Autodesk Inventor part; units mm, degrees
ref_plane "Work Plane1" through (-12.197, 0, 0) normal (0, -0.8660254, -0.5) x (1, 0, 0)
ref_plane "YZ Plane" through (0, 0, 0) normal (1, 0, 0) x (0, 1, 0)
ref_plane "XZ Plane" through (0, 0, 0) normal (0, 1, 0) x (-1, 0, 0)
sketch "Sketch1" plane through (0, 0, 0) normal (1, 0, 0) x (0, 1, 0)
  line L0 (-6.4231, 0) -> (-3.2116, 5.5626)
  line L1 (-3.2116, 5.5626) -> (3.2116, 5.5626)
  line L2 (3.2116, 5.5626) -> (6.4231, 0)
  line L3 (6.4231, 0) -> (3.2116, -5.5626)
  line L4 (3.2116, -5.5626) -> (-3.2116, -5.5626)
  line L5 (-3.2116, -5.5626) -> (-6.4231, 0)
  point P0 (0, 0)
  point P1 (0, 0)
  dimension "d0" = 12.8463
extrude "Body" add sketch "Sketch1" along normal blind 5.7404
sketch "Sketch2" plane through (0, 0, 0) normal (0, 0, 1) x (1, 0, 0)
  line L0 (0, 3.2116) -> (0, 6.4231)
  line L1 (0, 6.4231) -> (5.7404, 6.4231)
  line L2 (5.7404, 3.2116) -> (5.7404, 6.4231)
  line L3 (-1.1481, 0) -> (6.8885, 0)
  line L4 (0.4968, 6.4231) -> (0, 5.5626)
  line L5 (5.2436, 6.4231) -> (5.7404, 5.5626)
  dimension "d3" = 30
  dimension "d4" = 30
  dimension "d5" = 11.1252
  dimension "d6" = 11.1252
revolve "Chamfer1" cut sketch "Sketch2" angle 360 about axis through (-10, 0, 0) along (1, 0, 0)
sketch "Sketch3" plane through (5.7404, 0, 0) normal (1, 0, 0) x (0, 0, -1)
  arc A0 (-2.7813, -4.8174) -> (2.7813, -4.8174) centre (0, 0) ccw
hole "Thread" at (5.7404, 0, 0) direction (-1, 0, 0) diameter 4.9784 end through all
chamfer "Chamfer2" distance 0.6874 angle 30 1 edges at (5.7404, 0, 2.4892) measured on face at (5.7404, -4.5118, -0.1)
chamfer "Chamfer3" distance 0.6874 angle 30 1 edges at (0, 0, 2.4892) measured on face at (0, -4.5118, -0.1)
ref_plane "Work Plane1" through (-12.197, 0, 0) normal (0, -0.8660254, -0.5) x (1, 0, 0)
equation "\"d0\" = 1.1547 * SW"
equation "\"d1\" = KOH"
equation "\"d3\" = ANG1"
equation "\"d4\" = ANG2"
equation "\"d5\" = SW0"
equation "\"d6\" = SW01"
equation "\"d8\" = -0.5 * GD1 + 0.5 * NND"
equation "\"d40\" = -0.5 * GD1 + 0.5 * NND"
equation "\"d10\" = -0.5 * GD1 + 0.5 * NND"
equation "\"d41\" = -0.5 * GD1 + 0.5 * NND"
equation "\"ANG1\" = 30deg"
equation "\"ANG2\" = 30deg"
equation "\"NND\" = 6.35"
equation "\"KOH\" = 5.7404"
equation "\"SW\" = 11.1252"
equation "\"SW0\" = SW"
equation "\"SW01\" = SW"
equation "\"THREADDIA\" = 6.35"
equation "\"TOA\" = 30deg"
equation "\"E0\" = 1.155 * SW"
properties part number "AS 2465 - 1/4  UNC" material "Steel, Mild"
Read the model definition and answer for the solid it produces. Units are mm, in the model's axes. Coordinates: 2 decimals unless noted, no trailing zeros. Order: outer loops, then holes, each group sorted by start corner. A loop starts at its lowest first (then second) coordinate and runs counter-clockwise, first axis right, second up. Notation, with made-up numbers: (-40, -21) -> (-18, -21) arc R29 ccw to (-18, 11) -> close; hole circle Ø4 at (4, 47.25). An arc over 180 degrees is marked (long way). Answer as a JSON object with one key per item and string values.
1) A cutting plane is placed at A-A, the plane x = 3.8. Determine the outline of the cut face in (y, z), plus the area to 3 significant figures.
Model answer:
{"outline": "(-6.42, 0) -> (-3.21, -5.56) -> (3.21, -5.56) -> (6.42, 0) -> (3.21, 5.56) -> (-3.21, 5.56) -> close; hole circle Ø4.98 at (0, 0)", "area": "87.7 mm²"}
2) Each of these flat-tipped pins is pushed along its axis until it touches: pin 1 (1.5 mm diameter, centred on x = 3.5, z = 0.5, fed in from -Y); pin 2 (1.5 mm diameter, centred on x = 3, z = 4, fed in from +Y); pin 3 (1 mm diameter, centred on x = 2.5, z = -2.5, fed in from -Y). Where does it stop, or does it pass through?
Model answer:
{"pin 1": "stops at y = -6.42", "pin 2": "stops at y = 4.55", "pin 3": "stops at y = -5.27"}
3) Consider line 1 along Z through (x, y) = (3, 0); line 2 along Z through (x, y) = (1.1, 0.75); line 3 along Y through (x, z) = (3.8, -1.5). Determine where each line is inside the solid, lowest interval first. Write a range as from..to.
Model answer:
{"line 1": "z = -5.56..-2.49, 2.49..5.56", "line 2": "z = -5.56..-2.37, 2.37..5.56", "line 3": "y = -5.56..-1.99, 1.99..5.56"}
4) The mould has two halves that part along Y. Classify faces 1 (the face through (2.836, -0.748, -2.374)), 2 (the face through (2.83, 4.795, 2.82)), 3 (the face through (0.12, -2.87, 5.01)): released by +Y, released by -Y, zero draft, split by the parting line, or undercut.
Model answer:
{"face 1": "undercut", "face 2": "released by +Y", "face 3": "released by -Y"}
